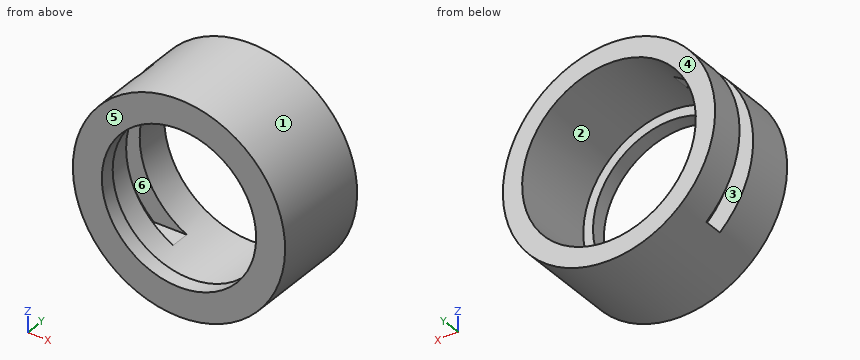
```python
from build123d import *

# Parameters (mm, degrees)
SKETCH2_W          = 80
SKETCH2_H          = 10
CUT_EXTRUDE1_DEPTH = 39


with BuildPart() as part:
    # Sketch1 → Revolve1 (revolve)
    with BuildSketch(Plane.XY, mode=Mode.PRIVATE) as revolve1_sk:
        Polygon((40, 7.915215599), (55, 7.915215599), (55, 60.915215599), (45, 60.915215599), (45, 15.915215599), (40, 15.915215599), align=None)
    revolve(revolve1_sk.sketch.rotate(Axis((0, 0, 0), (0, 1, 0)), 90), axis=Axis((0, 0, 0), (0, 1, 0)))

    # Sketch2 → Cut-Extrude1 (cut)
    with BuildSketch(Plane.ZY.offset(55)):
        with Locations((0, 37.915215599)):
            Rectangle(SKETCH2_W, SKETCH2_H)
    extrude(amount=-CUT_EXTRUDE1_DEPTH, mode=Mode.SUBTRACT)


solid = part.part
```
Geometry: final body of the model. Coordinates: model frame, mm. Face numbers are marked on the shaded views. A direction names the side the tool comes from. Round coordinates to 2 decimals unless told otherwise and drop trailing zeros. Write each loop counter-clockwise with the first axis right and the second up, starting at its lowest first coordinate (ties: lowest second). Pieces come first, ordered by that corner, then holes. Notation, with made-up numbers: (35.5, -21.75) -> (60.5, -21.75) arc R21 ccw to (60.5, -15.75) -> close; hole circle Ø4 at (-30, 88). An arc over 180 degrees is marked (long way). Return JSON: item names as keys, results as strings.
Q1. Set-up query: the marked faces 1, 2 and 3. Return all of +Z, -Z, +X, -X, +Y, -Y with unobstructed straight access to the full face (end or side cutting, diameter ignored); none if empty.
From the geometry:
{"face 1": "+Y, -Y", "face 2": "+Y", "face 3": "-X"}
Q2. Section A-A on x = 0. Return the cut outline in (y, z), and give its area (3 significant figures).
From the geometry:
{"outline": "(7.92, -55) -> (60.92, -55) -> (60.92, -45) -> (15.92, -45) -> (15.92, -40) -> (7.92, -40) -> close; (7.92, 40) -> (15.92, 40) -> (15.92, 45) -> (60.92, 45) -> (60.92, 55) -> (7.92, 55) -> close", "area": "1,140 mm2"}
Q3. Mould query, pull axis Y, two halves, no side actions, for the marked faces 4, 5 and 6. Classes: +Y half, -Y half, draft (parallel to the pull), parting line (faces both ways), or undercut.
From the geometry:
{"face 4": "+Y half", "face 5": "-Y half", "face 6": "undercut"}
Q4. Section C-C on y = 54. Return the cut outline in (x, z), and give its area (3 significant figures).
From the geometry:
{"outline": "circle Ø110 at (0, 0); hole circle Ø90 at (0, 0)", "area": "3,140 mm2"}
Q5. Section D-D on z = -27.5. Return the cut outline in (x, y).
From the geometry:
{"outline": "(-47.63, 7.92) -> (-29.05, 7.92) -> (-29.05, 15.92) -> (-35.62, 15.92) -> (-35.62, 32.92) -> (-47.63, 32.92) -> close; (-47.63, 42.92) -> (-35.62, 42.92) -> (-35.62, 60.92) -> (-47.63, 60.92) -> close; (29.05, 7.92) -> (47.63, 7.92) -> (47.63, 60.92) -> (35.62, 60.92) -> (35.62, 15.92) -> (29.05, 15.92) -> close"}
Q6. First-contact query: pin 1 Ø8 at (x, y) = (-31, 37) entering from -Z; pin 2 Ø3 at (x, y) = (16, 23) entering from +Z; pin 3 Ø3 at (x, y) = (-15, 24) entering from -Z; pin 4 Ø17 at (x, z) = (-39.5, 13.5) entering from +Y. Flat tips, straight axial feed; report the tip coordinate or a pass-through.
From the geometry:
{"pin 1": "z = -47.92", "pin 2": "z = 53.05", "pin 3": "z = -53.32", "pin 4": "y = 60.92"}
Q7. Ray query, line 1 (X direction, y = 31, z = 0); line 2 (Z direction, x = -8.5, y = 50.5); line 3 (X direction, y = 24, z = 32). Return the intervals inside material, ascending.
From the geometry:
{"line 1": "-55 to -45, 45 to 55", "line 2": "-54.34 to -44.19, 44.19 to 54.34", "line 3": "-44.73 to -31.64, 31.64 to 44.73"}
Q8. Section B-B on z = 0. Return the cut outline in (x, y).
From the geometry:
{"outline": "(-55, 7.92) -> (-40, 7.92) -> (-40, 15.92) -> (-45, 15.92) -> (-45, 32.92) -> (-55, 32.92) -> close; (-55, 42.92) -> (-45, 42.92) -> (-45, 60.92) -> (-55, 60.92) -> close; (40, 7.92) -> (55, 7.92) -> (55, 60.92) -> (45, 60.92) -> (45, 15.92) -> (40, 15.92) -> close"}
